```python
from build123d import *

# Parameters (mm, degrees)
BOSS_EXTRUDE1_DEPTH = 6.35
SKETCH4_W           = 71.12
SKETCH4_H           = 11.43
CUT_EXTRUDE1_DEPTH  = 258.233789577
SKETCH5_R           = 0.635
CUT_EXTRUDE2_DEPTH  = 258.233789577


with BuildPart() as part:
    # Sketch1 → Boss-Extrude1 (new body)
    with BuildSketch(Plane.XY):
        Polygon((215.9, 139.7), (215.9, -139.7), (117.222218475, -139.7), (0, 0), (117.222218475, 139.7), align=None)
    extrude(amount=BOSS_EXTRUDE1_DEPTH)

    # Sketch4 → Cut-Extrude1 (cut, through all)
    with BuildSketch(Plane.XY):
        with Locations((65.278, 0)):
            Rectangle(SKETCH4_W, SKETCH4_H)
    extrude(amount=CUT_EXTRUDE1_DEPTH, mode=Mode.SUBTRACT)

    # Sketch5 → Cut-Extrude2 (cut, through all)
    with BuildSketch(Plane.XY):
        with Locations((17.9578, 0)):
            Circle(SKETCH5_R)
        with Locations((119.5578, 0)):
            Circle(SKETCH5_R)
    extrude(amount=CUT_EXTRUDE2_DEPTH, mode=Mode.SUBTRACT)


solid = part.part
```
The listing builds one solid part. Answer for the finished solid, in the listing's coordinates (mm). A direction names the side the tool comes from. Give positions to 0.01 mm unless a question says otherwise; leave off trailing zeros. Order: outer loops, then holes, each group sorted by start corner. A loop starts at its lowest first (then second) coordinate and runs counter-clockwise, first axis right, second up. Notation, with made-up numbers: (68, -29) -> (116, -29) arc R20 cw to (116, -16) -> close; hole circle Ø5 at (4.5, -13.75). An arc over 180 degrees is marked (long way). Answer as a JSON object with one key per item and string values. Group by question number.
Item 1: The part is cut by section D-D on y = 14.5. Write down the section's boundary in (x, z), and give its area (3 significant figures).
Item 2: The part is cut by section C-C on x = 96. Write down the section's boundary in (y, z) (3 decimals), and give its area (3 significant figures).
Item 3: Flat-ended cylindrical pins translate along their axes: pin 1 (1 mm diameter, centred on x = 119.56, y = 0, fed in from +Z); pin 2 (1.9 mm diameter, centred on y = 0, z = 2.5, fed in from -X); pin 3 (1 mm diameter, centred on x = 66, z = 3.5, fed in from -Y); pin 4 (3 mm diameter, centred on x = 78.5, z = 4.5, fed in from +Y). Find the tip coordinate at first contact, or state that the pin passes through.
Item 4: The part is cut by section A-A on z = 2.5. Write down the section's boundary in (x, y) (3 decimals), and give its area (3 significant figures).
Item 5: A tool of negligible diameter and unlimited length cuts with its end or side. For faces 1 (the flat face through (29.718, 0, 3)), 2 (the flat face through (59.432, -70.828, 3.131)), from which of +Z, -Z, +X, -X, +Y, -Y can it reach the whole face along a straight path? Write none if from no direction.
Item 6: Determine the mould class of faces 3 (the flat face through (65, 5.715, 3)), 4 (the flat face through (166, 139.7, 3)), 5 (the flat face through (167, -139.7, 3)) for opening direction Y: pulls with the +Y half, pulls with the -Y half, needs draft (parallel to the pull), parting line crosses it, or undercut.
Item 7: Consider L1, parallel to X at y = 0, z = 4.75; L2, parallel to X at y = -3, z = 1.5; L3, parallel to X at y = 5.5, z = 0.5. Determine where each line is inside the solid, lowest interval first. Write a range as from..to.
Result set:
{
 "1": {"outline": "(12.17, 0) -> (215.9, 0) -> (215.9, 6.35) -> (12.17, 6.35) -> close", "area": "1,290 mm²"},
 "2": {"outline": "(-114.408, 0) -> (-5.715, 0) -> (-5.715, 6.35) -> (-114.408, 6.35) -> close; (5.715, 0) -> (114.408, 0) -> (114.408, 6.35) -> (5.715, 6.35) -> close", "area": "1,380 mm²"},
 "3": {"pin 1": "through", "pin 2": "x = 0", "pin 3": "y = -79.25", "pin 4": "y = 95.34"},
 "4": {"outline": "(0, 0) -> (117.222, -139.7) -> (215.9, -139.7) -> (215.9, 139.7) -> (117.222, 139.7) -> close; hole circle Ø1.27 at (17.958, 0); hole (29.718, -5.715) -> (100.838, -5.715) -> (100.838, 5.715) -> (29.718, 5.715) -> close; hole circle Ø1.27 at (119.558, 0)", "area": "43,100 mm²"},
 "5": {"face 1": "+Z, -Z", "face 2": "+Z, -Z, -X, -Y"},
 "6": {"face 3": "undercut", "face 4": "pulls with the +Y half", "face 5": "pulls with the -Y half"},
 "7": {"L1": "0..17.32, 18.59..29.72, 100.84..118.92, 120.19..215.9", "L2": "2.52..29.72, 100.84..215.9", "L3": "4.62..29.72, 100.84..215.9"}
}
